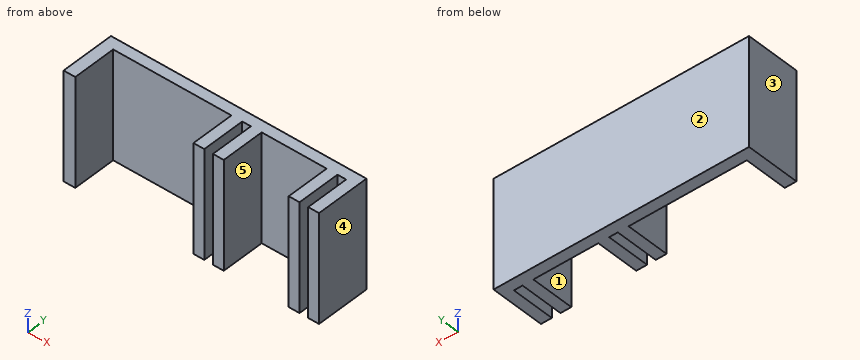
Autodesk Fusion 360 part; units mm, degrees
sketch "Sketch6" plane through (0, 0, 0) normal (0, 0, 1) x (1, 0, 0)
  line L0 (59, -2.5) -> (-59, -2.5)
  line L1 (-59, -2.5) -> (-59, 2.5)
  line L2 (-59, 2.5) -> (59, 2.5)
  line L3 (59, 2.5) -> (59, -2.5)
  line L4 (59, -2.5) -> (-59, 2.5) construction
  line L5 (-59, -2.5) -> (59, 2.5) construction
  dimension "d8" = 118
  dimension "d9" = 5
sketch "Sketch7" plane through (0, 0, 0) normal (0, 0, 1) x (1, 0, 0)
  line L0 (-464, -2.5) -> (-459, -2.5)
  line L1 (-459, -2.5) -> (-459, -22.5)
  line L2 (-459, -22.5) -> (-464, -22.5)
  line L3 (-464, -22.5) -> (-464, -2.5)
  line L4 (-459, -22.5) -> (-464, -22.5)
  line L5 (-464, -22.5) -> (-464, -2.5)
  line L6 (-459, -2.5) -> (-459, -22.5)
  line L7 (-464, -2.5) -> (-459, -2.5)
  dimension "d10" = 5
  dimension "d11" = 20
  dimension "d12" = 5
  dimension "d13" = 20
sketch "Sketch8" plane through (0, 0, 0) normal (0, 0, 1) x (1, 0, 0)
  line L0 (136, -2.5) -> (141, -2.5)
  line L1 (141, -2.5) -> (141, -22.5)
  line L2 (141, -22.5) -> (136, -22.5)
  line L3 (136, -22.5) -> (136, -2.5)
  dimension "d14" = 5
  dimension "d15" = 20
sketch "Sketch9" plane through (0, 0, 0) normal (0, 0, 1) x (1, 0, 0)
  line L0 (459, -2.5) -> (464, -2.5)
  line L1 (464, -2.5) -> (464, -22.5)
  line L2 (464, -22.5) -> (459, -22.5)
  line L3 (459, -22.5) -> (459, -2.5)
  dimension "d16" = 5
  dimension "d17" = 20
sketch "Sketch10" plane through (0, 0, 0) normal (0, 0, 1) x (1, 0, 0)
  line L0 (450, -2.5) -> (455, -2.5)
  line L1 (455, -2.5) -> (455, -22.5)
  line L2 (455, -22.5) -> (450, -22.5)
  line L3 (450, -22.5) -> (450, -2.5)
  dimension "d20" = 5
  dimension "d21" = 20
sketch "Sketch11" plane through (0, 0, 0) normal (0, 0, 1) x (1, 0, 0)
  line L0 (145, -2.5) -> (150, -2.5)
  line L1 (150, -2.5) -> (150, -22.5)
  line L2 (150, -22.5) -> (145, -22.5)
  line L3 (145, -22.5) -> (145, -2.5)
  dimension "d22" = 5
  dimension "d23" = 20
extrude "Extrude1" add sketch "Sketch6" along normal blind 100 makes body 1
extrude "Extrude2" add sketch "Sketch7" along normal blind 100 bodies 1 makes body 2
extrude "Extrude3" add sketch "Sketch8" along normal blind 100 bodies 2 makes body 3
extrude "Extrude4" add sketch "Sketch11" along normal blind 100 bodies 3 makes body 4
extrude "Extrude5" add sketch "Sketch10" along normal blind 100 bodies 4 makes body 5
extrude "Extrude6" add sketch "Sketch9" along normal blind 100 bodies 5 makes body 6
move_body "Move1" bodies 2 to x (1, 0, 0) y (0, 1, 0) z (0, 0, 1) at (418, 0, 0)
move_face "MoveFace1" by (-0.4, 0, 0) 1 faces at (-46, -15.8333, 33.3333) on bodies 2
move_body "Move2" bodies 5 6 to x (1, 0, 0) y (0, 1, 0) z (0, 0, 1) at (-417.6, 0, 0)
move_body "Move3" bodies 4 3 to x (1, 0, 0) y (0, 1, 0) z (0, 0, 1) at (-140, 0, 0)
move_body "Move4" bodies 3 4 to x (1, 0, 0) y (0, 1, 0) z (0, 0, 1) at (5, 0, 0)
move_body "Move5" bodies 4 3 to x (1, 0, 0) y (0, 1, 0) z (0, 0, 1) at (7, 0, 0)
move_body "Move6" bodies 4 3 to x (1, 0, 0) y (0, 1, 0) z (0, 0, 1) at (4, 0, 0)
move_body "Move7" bodies 2 to x (1, 0, 0) y (0, 1, 0) z (0, 0, 1) at (-12.6, 0, 0)
move_body "Move8" bodies 6 5 to x (1, 0, 0) y (0, 1, 0) z (0, 0, 1) at (12.6, 0, 0)
move_body "Move9" bodies 4 3 to x (1, 0, 0) y (0, 1, 0) z (0, 0, 1) at (-11, 0, 0)
combine "Combine1" operation add target body 1 tool bodies 2 3 4 6 5
extrude "Extrude7" cut 1 faces at (2, 0.8333, 100) along direction (0, 0, -1) blind 50 on bodies 1 bodies 1
Geometry: final body of the model. Coordinates: model frame, mm. Face numbers are marked on the shaded views. A direction names the side the tool comes from. Coordinates: 2 decimals unless noted, no trailing zeros. Order: outer loops, then holes, each group sorted by start corner. A loop starts at its lowest first (then second) coordinate and runs counter-clockwise, first axis right, second up.
1) Ray query, probe 1 along X at (y, z) = (-16.5, 7.5); probe 2 along Y at (x, z) = (30, 8). Return the intervals inside material, ascending.
Result sheet:
probe 1: x = -59 to -53.6, 1 to 6, 10 to 15, 45 to 50, 54 to 59
probe 2: y = -2.5 to 2.5
2) Section B-B (z = 42.5). Return loops of the section in (x, y), then the cut area to 3 significant figures.
Result sheet:
outline: (-59, -22.5) - (-53.6, -22.5) - (-53.6, -2.5) - (1, -2.5) - (1, -22.5) - (6, -22.5) - (6, -2.5) - (10, -2.5) - (10, -22.5) - (15, -22.5) - (15, -2.5) - (45, -2.5) - (45, -22.5) - (50, -22.5) - (50, -2.5) - (54, -2.5) - (54, -22.5) - (59, -22.5) - (59, 2.5) - (-59, 2.5) - close
area: 1,100 mm2
3) First-contact query: P1, Ø25, axis at x = -18.5, z = 31.5, coming from the -Y side. Flat tip, straight axial feed; report the tip coordinate or a pass-through.
Result sheet:
P1: stops at y = -2.5
4) Set-up query: the marked faces 4 and 5. Return all of +Z, -Z, +X, -X, +Y, -Y with unobstructed straight access to the full face (end or side cutting, diameter ignored); none if empty.
Result sheet:
face 4: +Z, -Z, +X, +Y, -Y
face 5: +Z, -Z, -Y
5) Section C-C (x = -40). Return loops of the section in (y, z).
Result sheet:
outline: (-2.5, 0) - (2.5, 0) - (2.5, 50) - (-2.5, 50) - close
6) Section A-A (y = -11.75). Return loops of the section in (x, z), then the cut area to 3 significant figures.
Result sheet:
outline: (-59, 0) - (-53.6, 0) - (-53.6, 50) - (-59, 50) - close; (1, 0) - (6, 0) - (6, 50) - (1, 50) - close; (10, 0) - (15, 0) - (15, 50) - (10, 50) - close; (45, 0) - (50, 0) - (50, 50) - (45, 50) - close; (54, 0) - (59, 0) - (59, 50) - (54, 50) - close
area: 1,270 mm2
7) Draft query along X for the marked faces 1, 2 and 3. Return one class per face: released by +X, released by -X, zero draft, split by the parting line, or undercut.
Result sheet:
face 1: undercut
face 2: zero draft
face 3: released by -X
